Geometry check sheet. Reference: the model listing, model coordinates, mm. A direction names the side the tool comes from. Round coordinates to 2 decimals unless told otherwise and drop trailing zeros. Write each loop counter-clockwise with the first axis right and the second up, starting at its lowest first coordinate (ties: lowest second). Pieces come first, ordered by that corner, then holes. Notation, with made-up numbers: (69.5, 23) -> (92.5, 23) arc R14 ccw to (92.5, 38) -> close; hole circle Ø5 at (17.5, 66). An arc over 180 degrees is marked (long way). Put each result on its own line as item: value. Start each with the question number.
from build123d import *

# Parameters (mm, degrees)
EXTRUDE_1_DEPTH     = 2.3
SKETCH_2_W          = 14
SKETCH_2_H          = 12.9
EXTRUDE_2_DEPTH     = 4.3
CUT_EXTRUDE_1_DEPTH = 27.297528401
SKETCH_4_W          = 14
SKETCH_4_H          = 13
EXTRUDE_3_DEPTH     = 12.2
FILLET_1_R          = 0.5
SKETCH_5_W          = 6
SKETCH_5_H          = 3
EXTRUDE_4_DEPTH     = 6.2
SKETCH_6_W          = 5
SKETCH_6_H          = 6.8
EXTRUDE_5_DEPTH     = 2.3
SKETCH_7_R          = 1.25
CUT_EXTRUDE_2_DEPTH = 33.607514471
FILLET_2_R          = 1.5
FILLET_3_R          = 0.3


with BuildPart() as part:
    # Эскиз1 → Бобышка-Вытянуть1 (new body)
    with BuildSketch(Plane.XY):
        with BuildLine():
            Line((1.5, 0), (16.5, 0))
            ThreePointArc((16.5, 0), (17.560660172, 0.439339828), (18, 1.5))
            Line((18, 1.5), (18, 16.5))
            ThreePointArc((18, 16.5), (17.560660172, 17.560660172), (16.5, 18))
            Line((16.5, 18), (1.5, 18))
            ThreePointArc((1.5, 18), (0.439339828, 17.560660172), (0, 16.5))
            Line((0, 16.5), (0, 1.5))
            ThreePointArc((0, 1.5), (0.439339828, 0.439339828), (1.5, 0))
        make_face()
    extrude(amount=EXTRUDE_1_DEPTH)

    # Эскиз2 → Бобышка-Вытянуть2 (add)
    with BuildSketch(Plane(origin=(0, 0, 0), x_dir=(-1, 0, 0), z_dir=(0, 0, -1))):
        with Locations((-9, 9)):
            Rectangle(SKETCH_2_W, SKETCH_2_H)
    extrude(amount=EXTRUDE_2_DEPTH)

    # Эскиз3 → Вырез-Вытянуть1 (cut, through all)
    with BuildSketch(Plane(origin=(0, 0, -4.3), x_dir=(-1, 0, 0), z_dir=(0, 0, -1))):
        Polygon((-14.5, 12.55), (-12.83154497, 13.95), (-5.16845503, 13.95), (-3.5, 12.55), (-3.5, 4.05), (-14.5, 4.05), align=None)
    extrude(amount=-CUT_EXTRUDE_1_DEPTH, mode=Mode.SUBTRACT)

    # Эскиз4 → Бобышка-Вытянуть3 (add)
    with BuildSketch(Plane.XY.offset(2.3)):
        with Locations((9, 9)):
            Rectangle(SKETCH_4_W, SKETCH_4_H)
    extrude(amount=EXTRUDE_3_DEPTH)

    # Скругление1
    fillet_1_edges = [part.edges().sort_by_distance(p)[0] for p in [
        (16, 15.45, -2.15),
        (16, 2.55, -2.15),
        (2, 2.55, -2.15),
        (2, 15.45, -2.15),
        (2, 15.5, 8.4),
        (2, 2.5, 8.4),
        (16, 2.5, 8.4),
        (16, 15.5, 8.4),
    ]]
    fillet(fillet_1_edges, radius=FILLET_1_R)

    # Эскиз5 → Бобышка-Вытянуть4 (add)
    with BuildSketch(Plane(origin=(0, 0, 2.3), x_dir=(-1, 0, 0), z_dir=(0, 0, -1))):
        with Locations((-9, 9)):
            Rectangle(SKETCH_5_W, SKETCH_5_H)
    extrude(amount=EXTRUDE_4_DEPTH)

    # Эскиз6 → Бобышка-Вытянуть5 (add)
    with BuildSketch(Plane(origin=(0, 0, 0), x_dir=(-1, 0, 0), z_dir=(0, 0, -1))):
        with Locations((-20.5, 9)):
            Rectangle(SKETCH_6_W, SKETCH_6_H)
        with Locations((2.5, 9)):
            Rectangle(SKETCH_6_W, SKETCH_6_H)
    extrude(amount=-EXTRUDE_5_DEPTH)

    # Эскиз7 → Вырез-Вытянуть2 (cut, through all)
    with BuildSketch(Plane(origin=(0, 0, 0), x_dir=(-1, 0, 0), z_dir=(0, 0, -1))):
        with Locations((-20, 9)):
            Circle(SKETCH_7_R)
        with Locations((2, 9)):
            Circle(SKETCH_7_R)
    extrude(amount=-CUT_EXTRUDE_2_DEPTH, mode=Mode.SUBTRACT)

    # Скругление2
    fillet_2_edges = [part.edges().sort_by_distance(p)[0] for p in [
        (18, 12.4, 1.15),
        (18, 5.6, 1.15),
        (23, 5.6, 1.15),
        (23, 12.4, 1.15),
        (0, 5.6, 1.15),
        (0, 12.4, 1.15),
        (-5, 12.4, 1.15),
        (-5, 5.6, 1.15),
    ]]
    fillet(fillet_2_edges, radius=FILLET_2_R)

    # Скругление3
    fillet_3_edges = [part.edges().sort_by_distance(p)[0] for p in [
        (12, 10.5, -0.8),
        (12, 7.5, -0.8),
        (6, 7.5, -0.8),
        (6, 10.5, -0.8),
    ]]
    fillet(fillet_3_edges, radius=FILLET_3_R)


solid = part.part
(1) Sectioned sample at C-C (y = 9). Record the cut outline in (x, z).
(2) Sectioned sample at B-B (z = -3). Record the cut outline in (x, y).
(3) Sectioned sample at A-A (x = 20). Record the cut outline in (y, z).
(4) Go/stop test with flat-tipped pins: pin 1 Ø0.7 at (y, z) = (9, -1) entering from -X; pin 2 Ø1.8 at (y, z) = (15, 1.5) entering from -X; pin 3 Ø3 at (x, y) = (11.5, 8) entering from -Z. Record where each tip stops, or that it passes through.
(5) Sectioned sample at D-D (x = 6.75). Record the cut outline in (y, z), and give its area (3 significant figures).
(6) Material ranges on L1, parallel to Y at x = 10, z = -2.5; L2, parallel to Y at x = 9, z = 1; L3, parallel to Y at x = 20, z = 1.4, recorded low to high. Write a range as from..to.
(7) Mould release check, pull along X, two halves, no side actions. Record for faces 4 (the flat face through (9, 10.5, -1)), 5 (the cylindrical face through (-0.43, 5.15, 1.17)), 6 (the flat face through (9, 7, 2.3)), 7 (the flat face through (9, 18, 1)): +X half, -X half, draft (parallel to the pull), parting line (faces both ways), or undercut.
(8) Set-up check for faces 1 (the flat face through (9, 7.5, -1)), 2 (the flat face through (18, 15, 1)), 3 (the flat face through (9, 15.45, -2)): record each of +Z, -Z, +X, -X, +Y, -Y from which the full face is reachable in a straight line by a thin tool's end or side.
Found:
1. outline: (-5, 0) -> (-3.25, 0) -> (-3.25, 2.3) -> (-5, 2.3) -> close; (-0.75, 0) -> (2, 0) -> (2, -4.3) -> (3.5, -4.3) -> (3.5, 2.3) -> (6, 2.3) -> (6, -3.9) -> (12, -3.9) -> (12, 2.3) -> (14.5, 2.3) -> (14.5, -4.3) -> (16, -4.3) -> (16, 0) -> (18.75, 0) -> (18.75, 2.3) -> (16, 2.3) -> (16, 14.5) -> (2, 14.5) -> (2, 2.3) -> (-0.75, 2.3) -> close; (21.25, 0) -> (23, 0) -> (23, 2.3) -> (21.25, 2.3) -> close
2. outline: (2, 3.05) arc R0.5 ccw to (2.5, 2.55) -> (15.5, 2.55) arc R0.5 ccw to (16, 3.05) -> (16, 14.95) arc R0.5 ccw to (15.5, 15.45) -> (2.5, 15.45) arc R0.5 ccw to (2, 14.95) -> close; (6, 7.8) arc R0.3 ccw to (6.3, 7.5) -> (11.7, 7.5) arc R0.3 ccw to (12, 7.8) -> (12, 10.2) arc R0.3 ccw to (11.7, 10.5) -> (6.3, 10.5) arc R0.3 ccw to (6, 10.2) -> close; hole (3.5, 4.05) -> (14.5, 4.05) -> (14.5, 12.55) -> (12.83, 13.95) -> (5.17, 13.95) -> (3.5, 12.55) -> close
3. outline: (5.6, 0) -> (7.75, 0) -> (7.75, 2.3) -> (5.6, 2.3) -> close; (10.25, 0) -> (12.4, 0) -> (12.4, 2.3) -> (10.25, 2.3) -> close
4. pin 1: x = 2
4. pin 2: x = 0
4. pin 3: z = -3.9
5. outline: (0, 0) -> (2.55, 0) -> (2.55, -4.3) -> (4.05, -4.3) -> (4.05, 2.3) -> (7.5, 2.3) -> (7.5, -3.9) -> (10.5, -3.9) -> (10.5, 2.3) -> (13.95, 2.3) -> (13.95, -4.3) -> (15.45, -4.3) -> (15.45, 0) -> (18, 0) -> (18, 2.3) -> (15.5, 2.3) -> (15.5, 14.5) -> (2.5, 14.5) -> (2.5, 2.3) -> (0, 2.3) -> close
5. area: 209 mm2
6. L1: 2.55..4.05, 7.5..10.5, 13.95..15.45
6. L2: 0..4.05, 7.5..10.5, 13.95..18
6. L3: 5.6..7.75, 10.25..12.4
7. face 4: undercut
7. face 5: -X half
7. face 6: undercut
7. face 7: draft
8. face 1: -Z
8. face 2: +Z, -Z, +X, +Y
8. face 3: -Z, +X, -X, +Y
